from build123d import *

# Parameters (mm, degrees)
F2_R        = 1.75
F3_DEPTH    = 6.5
F4_R        = 2.75
F5_DEPTH    = 3.5
F6_T1_DEPTH = 57.2838374918
F6_T3_DEPTH = 62.3332762367
F6_T5_DEPTH = 62.0777502529
F7_R        = 3.25
F8_DEPTH    = 4


# Not quite as in the source:
# - a fillet or chamfer that OpenCascade refuses, or shapes differently, is made with other operations: its cross-section is extruded or revolved along the edge and cut away or added


with BuildPart() as f3:
    # F2 (on Top) → F3 (new body)
    with BuildSketch(Plane.XY):
        with BuildLine():
            ThreePointArc((-3.1189043715, 2.8870288397), (-1.7018559621, 3.894378806), (0, 4.25))
            ThreePointArc((0, 4.25), (1.6264045876, 3.9264880132), (3.00520382, 3.00520382))
            Line((3.00520382, 3.00520382), (5.5861435714, 5.5861435714))
            ThreePointArc((5.5861435714, 5.5861435714), (5.5861435714, 7.8488852712), (7.8488852712, 7.8488852712))
            Line((7.8488852712, 7.8488852712), (10.0716416635, 10.0716416635))
            ThreePointArc((10.0716416635, 10.0716416635), (8.0706751581, 14.271751719), (9.6732808742, 18.6394108579))
            ThreePointArc((9.6732808742, 18.6394108579), (-0.2919239613, 20.9979708639), (-10.1877103957, 18.3632937376))
            ThreePointArc((-10.1877103957, 18.3632937376), (-9.2786875084, 16.6483019778), (-8.9647275629, 14.732852031))
            ThreePointArc((-8.9647275629, 14.732852031), (-9.4214503678, 12.4367514369), (-10.7220868758, 10.4902113439))
            Line((-10.7220868758, 10.4902113439), (-6.9029746628, 6.6710991309))
            ThreePointArc((-6.9029746628, 6.6710991309), (-5.1593103211, 7.017935533), (-4.1716038129, 5.539728281))
            ThreePointArc((-4.1716038129, 5.539728281), (-4.2933965608, 4.9274347892), (-4.640232963, 4.4083574311))
            Line((-4.640232963, 4.4083574311), (-3.1189043715, 2.8870288397))
        make_face()
        with BuildLine():
            ThreePointArc((0, 14.5134559673), (-1.2374368671, 17.5008928344), (1.75, 16.2634559673))
            ThreePointArc((1.75, 16.2634559673), (1.2374368671, 15.0260191002), (0, 14.5134559673))
        make_face(mode=Mode.SUBTRACT)
        with BuildLine():
            ThreePointArc((-4.25, 0), (-3.9571355536, 1.5503477708), (-3.1189043715, 2.8870288397))
            Line((-3.1189043715, 2.8870288397), (-4.640232963, 4.4083574311))
            ThreePointArc((-4.640232963, 4.4083574311), (-6.9029746628, 4.4083574311), (-6.9029746628, 6.6710991309))
            Line((-6.9029746628, 6.6710991309), (-10.7220868758, 10.4902113439))
            ThreePointArc((-10.7220868758, 10.4902113439), (-14.5116932272, 8.7499798202), (-18.5201343168, 9.899728526))
            ThreePointArc((-18.5201343168, 9.899728526), (-20.9996146914, 0.1272116798), (-18.6387120488, -9.674627288))
            ThreePointArc((-18.6387120488, -9.674627288), (-14.279821029, -8.0983145468), (-10.0983841523, -10.0983841523))
            Line((-10.0983841523, -10.0983841523), (-7.8488852712, -7.8488852712))
            ThreePointArc((-7.8488852712, -7.8488852712), (-7.8488852712, -5.5861435714), (-5.5861435714, -5.5861435714))
            Line((-5.5861435714, -5.5861435714), (-3.00520382, -3.00520382))
            ThreePointArc((-3.00520382, -3.00520382), (-3.9264880132, -1.6264045876), (-4.25, 0))
        make_face()
        with Locations((-16.2634559673, 0)):
            Circle(F2_R, mode=Mode.SUBTRACT)
        with BuildLine():
            Line((5.5861435714, 5.5861435714), (3.00520382, 3.00520382))
            ThreePointArc((3.00520382, 3.00520382), (3.9264880132, 1.6264045876), (4.25, 0))
            ThreePointArc((4.25, 0), (3.894378806, -1.7018559621), (2.8870288397, -3.1189043715))
            Line((2.8870288397, -3.1189043715), (4.4083574311, -4.640232963))
            ThreePointArc((4.4083574311, -4.640232963), (6.1520217728, -4.2933965608), (7.139728281, -5.7716038129))
            ThreePointArc((7.139728281, -5.7716038129), (7.017935533, -6.3838973046), (6.6710991309, -6.9029746628))
            Line((6.6710991309, -6.9029746628), (10.4902113439, -10.7220868758))
            ThreePointArc((10.4902113439, -10.7220868758), (14.3265437078, -8.9785005753), (18.3632937376, -10.1877103957))
            ThreePointArc((18.3632937376, -10.1877103957), (20.3301397989, -5.2616932403), (21, 0))
            ThreePointArc((21, 0), (20.3137902, 5.3244650163), (18.3000068848, 10.3009585969))
            ThreePointArc((18.3000068848, 10.3009585969), (14.2313497781, 8.552751018), (10.0716416635, 10.0716416635))
            Line((10.0716416635, 10.0716416635), (7.8488852712, 7.8488852712))
            ThreePointArc((7.8488852712, 7.8488852712), (8.1957216733, 7.3298079131), (8.3175144213, 6.7175144213))
            ThreePointArc((8.3175144213, 6.7175144213), (7.3298079131, 5.2393071693), (5.5861435714, 5.5861435714))
        make_face()
        with BuildLine():
            ThreePointArc((18.0134559673, 0), (16.2634559673, -1.75), (14.5134559673, 0))
            ThreePointArc((14.5134559673, 0), (16.2634559673, 1.75), (18.0134559673, 0))
        make_face(mode=Mode.SUBTRACT)
        with BuildLine():
            Line((4.4083574311, -4.640232963), (2.8870288397, -3.1189043715))
            ThreePointArc((2.8870288397, -3.1189043715), (1.5503477708, -3.9571355536), (0, -4.25))
            ThreePointArc((0, -4.25), (-1.6264045876, -3.9264880132), (-3.00520382, -3.00520382))
            Line((-3.00520382, -3.00520382), (-5.5861435714, -5.5861435714))
            ThreePointArc((-5.5861435714, -5.5861435714), (-5.2393071693, -6.1052209295), (-5.1175144213, -6.7175144213))
            ThreePointArc((-5.1175144213, -6.7175144213), (-6.1052209295, -8.1957216733), (-7.8488852712, -7.8488852712))
            Line((-7.8488852712, -7.8488852712), (-10.0983841523, -10.0983841523))
            ThreePointArc((-10.0983841523, -10.0983841523), (-8.9703530251, -11.9546705323), (-8.577165246, -14.0909422189))
            ThreePointArc((-8.577165246, -14.0909422189), (-9.024856678, -16.365116699), (-10.301121768, -18.2999150359))
            ThreePointArc((-10.301121768, -18.2999150359), (-0.2289175978, -20.9987522661), (9.899728526, -18.5201343168))
            ThreePointArc((9.899728526, -18.5201343168), (8.7499798202, -14.5116932272), (10.4902113439, -10.7220868758))
            Line((10.4902113439, -10.7220868758), (6.6710991309, -6.9029746628))
            ThreePointArc((6.6710991309, -6.9029746628), (4.4083574311, -6.9029746628), (4.4083574311, -4.640232963))
        make_face()
        with BuildLine():
            ThreePointArc((1.75, -16.2634559673), (-1.2374368671, -17.5008928344), (0, -14.5134559673))
            ThreePointArc((0, -14.5134559673), (1.2374368671, -15.0260191002), (1.75, -16.2634559673))
        make_face(mode=Mode.SUBTRACT)
    extrude(amount=F3_DEPTH)

    # F4 (on face) → F5 (cut)
    with BuildSketch(Plane.XY.offset(6.5)):
        with Locations((-5.7716038129, 5.539728281)):
            Circle(F4_R)
        with Locations((5.539728281, -5.7716038129)):
            Circle(F4_R)
        with Locations((-6.7175144213, -6.7175144213)):
            Circle(F4_R)
        with Locations((6.7175144213, 6.7175144213)):
            Circle(F4_R)
    extrude(amount=-F5_DEPTH, mode=Mode.SUBTRACT)

    # F6: fillet of radius 9 on 8 edges, made by hand

    # F6_s2 → F6_t1 (cut)
    with BuildSketch(Plane.XY.offset(-25.3919187459)):
        with BuildLine():
            ThreePointArc((-0.3782425644, 20.9965933561), (-6.0328802021, 18.8657689221), (-9.065291981, 13.6389325572))
            ThreePointArc((-9.065291981, 13.6389325572), (-9.1272145679, 16.1197341578), (-10.1877103957, 18.3632937376))
            ThreePointArc((-10.1877103957, 18.3632937376), (-5.4445759439, 20.2819277385), (-0.3782425644, 20.9965933561))
        make_face()
        with BuildLine():
            ThreePointArc((20.9965933561, -0.3782425644), (18.8657689221, -6.0328802021), (13.6389325572, -9.065291981))
            ThreePointArc((13.6389325572, -9.065291981), (16.1197341578, -9.1272145679), (18.3632937376, -10.1877103957))
            ThreePointArc((18.3632937376, -10.1877103957), (20.2819277385, -5.4445759439), (20.9965933561, -0.3782425644))
        make_face()
        with BuildLine():
            ThreePointArc((-13.7788227476, 8.8512170739), (-18.9576712537, 5.7375588181), (-20.9999396683, 0.0503381168))
            ThreePointArc((-20.9999396683, 0.0503381168), (-20.3644711398, 5.1272131997), (-18.5201343168, 9.899728526))
            ThreePointArc((-18.5201343168, 9.899728526), (-16.2602888025, 8.8743948046), (-13.7788227476, 8.8512170739))
        make_face()
        with BuildLine():
            ThreePointArc((0.0503381168, -20.9999396683), (5.7375588181, -18.9576712537), (8.8512170739, -13.7788227476))
            ThreePointArc((8.8512170739, -13.7788227476), (8.8743948046, -16.2602888025), (9.899728526, -18.5201343168))
            ThreePointArc((9.899728526, -18.5201343168), (5.1272131997, -20.3644711398), (0.0503381168, -20.9999396683))
        make_face()
    extrude(amount=F6_T1_DEPTH, mode=Mode.SUBTRACT)

    # F6_s4 → F6_t3 (cut)
    with BuildSketch(Plane.XY.offset(-27.9166381183)):
        with BuildLine():
            ThreePointArc((-1.2489870314, 20.962824986), (4.8716041748, 19.0359733336), (8.1530373835, 13.5217562449))
            ThreePointArc((8.1530373835, 13.5217562449), (8.3126072664, 16.2589826676), (9.6732808742, 18.6394108579))
            ThreePointArc((9.6732808742, 18.6394108579), (4.3694101421, 20.5404054247), (-1.2489870314, 20.962824986))
        make_face()
        with BuildLine():
            ThreePointArc((13.2369559696, 8.6077236934), (18.8594743215, 5.515526839), (20.993156783, -0.5360674268))
            ThreePointArc((20.993156783, -0.5360674268), (20.3800996321, 5.0647348385), (18.3000068848, 10.3009585969))
            ThreePointArc((18.3000068848, 10.3009585969), (15.9671809198, 8.8601969743), (13.2369559696, 8.6077236934))
        make_face()
    extrude(amount=F6_T3_DEPTH, mode=Mode.SUBTRACT)

    # F6_s6 → F6_t5 (cut)
    with BuildSketch(Plane.XY.offset(-27.7888751265)):
        with BuildLine():
            ThreePointArc((-8.6359238746, -13.2532961322), (-5.5485972344, -18.85793385), (0.4828918194, -20.9944472538))
            ThreePointArc((0.4828918194, -20.9944472538), (-5.090632161, -20.3736463158), (-10.301121768, -18.2999150359))
            ThreePointArc((-10.301121768, -18.2999150359), (-8.8793307439, -15.9710172139), (-8.6359238746, -13.2532961322))
        make_face()
        with BuildLine():
            ThreePointArc((-20.9659970002, 1.1945584074), (-19.0352466943, -4.9059131307), (-13.5385270334, -8.1815234096))
            ThreePointArc((-13.5385270334, -8.1815234096), (-16.2629392178, -8.3326294351), (-18.6387120488, -9.674627288))
            ThreePointArc((-18.6387120488, -9.674627288), (-20.5345573153, -4.3968120117), (-20.9659970002, 1.1945584074))
        make_face()
    extrude(amount=F6_T5_DEPTH, mode=Mode.SUBTRACT)

    # F7 (on face) → F8 (cut)
    with BuildSketch(Plane.XY.offset(6.5)):
        with Locations((-16.2634559673, 0)):
            Circle(F7_R)
        with Locations((0, 16.2634559673)):
            Circle(F7_R)
        with Locations((16.2634559673, 0)):
            Circle(F7_R)
        with Locations((0, -16.2634559673)):
            Circle(F7_R)
    extrude(amount=-F8_DEPTH, mode=Mode.SUBTRACT)


solid = f3.part
Design review of the part built by this model. Coordinates are the model's own, in mm. A direction names the side the tool comes from. Give positions to 0.01 mm unless a question says otherwise; leave off trailing zeros. Order: outer loops, then holes, each group sorted by start corner. A loop starts at its lowest first (then second) coordinate and runs counter-clockwise, first axis right, second up.
1. Mouldability with a two-part tool opening along Y and no side actions: class faces 3 (the cylindrical face through (7.018, -3.453, 4.774)), 4 (the cylindrical face through (-5.698, -18.728, 3.205)), 5 (the cylindrical face through (-6.13, 18.78, 3.2)) as +Y half, -Y half, draft (parallel to the pull), parting line (faces both ways), or undercut.
Solution:
face 3: undercut
face 4: -Y half
face 5: +Y half
2. To check wall thickness, follow L1, parallel to X at y = -6, z = 5; L2, parallel to X at y = 3.5, z = 5.5; L3, parallel to X at y = -1.5, z = 2. State the ranges of each line that lie inside material, in increasing order.
Solution:
L1: x = -18.01 to -9.37, -4.06 to 2.8, 8.28 to 18.89
L2: x = -20.3 to -7.62, -3.93 to -2.41, 2.41 to 20.15
L3: x = -20.71 to -17.16, -15.36 to -3.98, 3.98 to 15.36, 17.16 to 20.91
3. For pin 1 Ø1 at (x, z) = (10.5, 4.5) entering from +Y; pin 2 Ø4.5 at (x, y) = (-16.26, 0) entering from -Z; pin 3 Ø3 at (x, y) = (0, 16.26) entering from -Z; pin 4 Ø6 at (x, y) = (0, -16.26) entering from +Z, all flat-tipped, find the tip position at first contact; note any pin that passes through.
Solution:
pin 1: stops at y = 10.14
pin 2: stops at z = 0
pin 3: passes through
pin 4: stops at z = 2.5
4. Add section C-C, the plane y = 12. State the section outline as (x, z) points.
Solution:
outline: (-9.62, 0) - (8.63, 0) - (8.63, 6.5) - (-9.62, 6.5) - close
5. Add section B-B, the plane x = -12.5. State the section outline as (y, z) points.
Solution:
outline: (-8.46, 0) - (9.26, 0) - (9.26, 6.5) - (-8.46, 6.5) - close
6. Add section A-A, the plane z = 6. State how many separate pieces and enclosed holes the cut face has, then the cut area to 3 significant figures.
Solution:
separate pieces: 1
enclosed holes: 9
area: 768 mm2
7. Tool access review of faces 1 (the cylindrical face through (19.363, 0.976, 4.528)), 2 (the cylindrical face through (14.594, 0.526, 1.232)): name each direction out of +Z, -Z, +X, -X, +Y, -Y from which nothing blocks a thin tool from reaching the whole face with its end or side.
Solution:
face 1: +Z
face 2: +Z, -Z
